```python
from build123d import *

# Parameters (mm, degrees)
SKETCH2_W                        = 90
SKETCH2_H                        = 90
BOSS_EXTRUDE1_DEPTH              = 103
SKETCH4_W                        = 24
SKETCH4_H                        = 25
SKETCH4_W_2                      = 40
SKETCH4_H_2                      = 17.5
SKETCH4_W_3                      = 3
SKETCH4_H_3                      = 4
SKETCH5_R                        = 10
CUT_EXTRUDE1_DEPTH               = 46
CUT_EXTRUDE1_DEPTH_BACK          = 46
SKETCH6_W                        = 87.169413833
SKETCH6_H                        = 43.101198191
CUT_EXTRUDE2_DEPTH               = 46
CUT_EXTRUDE2_DEPTH_BACK          = 46
CUT_EXTRUDE3_DEPTH               = 103
CUT_EXTRUDE4_REACH               = 92
SKETCH10_R                       = 1.7
FILLET1_R                        = 1
M16X1_5_TAPPED_HOLE2_D           = 14.5
M16X1_5_TAPPED_HOLE2_DEPTH       = 20
M16X1_5_TAPPED_HOLE2_CSINK_D     = 16.05
M16X1_5_TAPPED_HOLE2_CSINK_ANGLE = 90
M16X1_5_TAPPED_HOLE2_TIP         = 4.356239488
CIRPATTERN2_COUNT                = 4


with BuildPart() as part:
    # Sketch2 → Boss-Extrude1 (new body)
    with BuildSketch(Plane.XY):
        Rectangle(SKETCH2_W, SKETCH2_H)
    extrude(amount=BOSS_EXTRUDE1_DEPTH)

    # Sketch4 → Cut-Revolve2 (revolve, cut)
    with BuildSketch(Plane(origin=(0, 0, 0), x_dir=(1, 0, 0), z_dir=(0, 1, 0))):
        with Locations((12, -12.5)):
            Rectangle(SKETCH4_W, SKETCH4_H)
        Polygon((0, -25), (0, -39.420654857), (24, -25), align=None)
        with Locations((50, -8.75)):
            Rectangle(SKETCH4_W_2, SKETCH4_H_2)
        with Locations((28.5, -4.5)):
            Rectangle(SKETCH4_W_3, SKETCH4_H_3)
    revolve(axis=Axis((0, 0, 0), (0, 0, 1)), mode=Mode.SUBTRACT)

    # Sketch5 → Cut-Extrude1 (cut, two sides)
    with BuildSketch(Plane(origin=(0, 0, 0), x_dir=(0, 0, -1), z_dir=(1, 0, 0))) as cut_extrude1_sk:
        with Locations((-77.5, 0)):
            Circle(SKETCH5_R)
    extrude(amount=CUT_EXTRUDE1_DEPTH, mode=Mode.SUBTRACT)
    extrude(cut_extrude1_sk.sketch, amount=-CUT_EXTRUDE1_DEPTH_BACK, mode=Mode.SUBTRACT)

    # Sketch6 → Cut-Revolve3 (revolve, cut)
    with BuildSketch(Plane(origin=(0, 0, 0), x_dir=(0, 0, -1), z_dir=(1, 0, 0))):
        with Locations((-91.084706917, 51.550599096)):
            Rectangle(SKETCH6_W, SKETCH6_H)
    revolve(axis=Axis((0, 0, 0), (0, 0, 1)), mode=Mode.SUBTRACT)

    # Sketch7 → Cut-Extrude2 (cut, two sides)
    with BuildSketch(Plane(origin=(0, 0, 0), x_dir=(0, 0, -1), z_dir=(1, 0, 0))) as cut_extrude2_sk:
        with BuildLine():
            Line((-103, 30), (-103, 0))
            ThreePointArc((-103, 0), (-95.748626332, 19.557607216), (-77.5, 29.6605799))
            Line((-77.5, 29.6605799), (-77.5, 30))
            Line((-77.5, 30), (-103, 30))
        make_face()
        with BuildLine():
            ThreePointArc((-77.5, -29.6605799), (-95.748626332, -19.557607216), (-103, 0))
            Line((-103, 0), (-103, -30))
            Line((-103, -30), (-77.5, -30))
            Line((-77.5, -30), (-77.5, -29.6605799))
        make_face()
    extrude(amount=CUT_EXTRUDE2_DEPTH, mode=Mode.SUBTRACT)
    extrude(cut_extrude2_sk.sketch, amount=-CUT_EXTRUDE2_DEPTH_BACK, mode=Mode.SUBTRACT)

    # Sketch8 → Cut-Extrude3 (cut)
    with BuildSketch(Plane.XY.offset(47.5)):
        with BuildLine():
            ThreePointArc((30, 0), (28.722813233, 8.660254038), (25, 16.583123952))
            Line((25, 16.583123952), (25, -16.583123952))
            ThreePointArc((25, -16.583123952), (28.722813233, -8.660254038), (30, 0))
        make_face()
        with BuildLine():
            Line((-25, -16.583123952), (-25, 16.583123952))
            ThreePointArc((-25, 16.583123952), (-30, 0), (-25, -16.583123952))
        make_face()
        with BuildLine():
            ThreePointArc((10, 28.284271247), (0, 30), (-10, 28.284271247))
            Line((-10, 28.284271247), (-10, -28.284271247))
            ThreePointArc((-10, -28.284271247), (0, -30), (10, -28.284271247))
            Line((10, -28.284271247), (10, 28.284271247))
        make_face()
    extrude(amount=CUT_EXTRUDE3_DEPTH, mode=Mode.SUBTRACT)

    # Sketch10 → Cut-Extrude4 (cut, up to next)
    with BuildSketch(Plane(origin=(0, 45, 0), x_dir=(1, 0, 0), z_dir=(0, 1, 0)), mode=Mode.PRIVATE) as cut_extrude4_sk1:
        with Locations((0, -32.5)):
            Circle(SKETCH10_R)
    cut_extrude4_tool1 = extrude(cut_extrude4_sk1.sketch, amount=-CUT_EXTRUDE4_REACH, mode=Mode.PRIVATE) & part.part
    add(cut_extrude4_tool1.solids().sort_by_distance((0, 45, 32.5))[0], mode=Mode.SUBTRACT)

    # Fillet1
    fillet1_edges = [part.edges().sort_by_distance(p)[0] for p in [
        (18.452078799, 23.654191764, 47.5),
        (18.452078799, -23.654191764, 47.5),
        (-18.452078799, -23.654191764, 47.5),
        (25, 0, 47.5),
        (-25, 0, 47.5),
        (-10, 0, 47.5),
        (10, 0, 47.5),
        (-30, 0, 17.5),
        (-18.452078799, 23.654191764, 47.5),
    ]]
    fillet(fillet1_edges, radius=FILLET1_R)

    # M16x1.5 Tapped Hole2
    with Locations(Plane(origin=(0, 45, 0), x_dir=(1, 0, 0), z_dir=(0, 1, 0))):
        with Locations((0, -32.5)):
            CounterSinkHole(M16X1_5_TAPPED_HOLE2_D / 2, M16X1_5_TAPPED_HOLE2_CSINK_D / 2, depth=M16X1_5_TAPPED_HOLE2_DEPTH, counter_sink_angle=M16X1_5_TAPPED_HOLE2_CSINK_ANGLE)
            with Locations((0, 0, -(M16X1_5_TAPPED_HOLE2_DEPTH + M16X1_5_TAPPED_HOLE2_TIP / 2))):  # 118° drill point
                Cone(0, M16X1_5_TAPPED_HOLE2_D / 2, M16X1_5_TAPPED_HOLE2_TIP, mode=Mode.SUBTRACT)

    # Sketch25 → M12x1.5 Tapped Hole1 (revolve, cut)
    with BuildSketch(Plane(origin=(31.819805153, 31.819805153, 17.5), x_dir=(0, 1, 0), z_dir=(1, 0, 0))):
        Polygon((0, 0), (0, 23.15451825), (5.25, 20), (5.25, 0.775), (6.025, 0), align=None)
    m12x1_5_tapped_hole1 = revolve(axis=Axis((31.819805153, 31.819805153, 11.15), (0, 0, 1)), mode=Mode.SUBTRACT)

    # CirPattern2: M12x1.5 Tapped Hole1 ×4 about axis
    cirpattern2_axis = Axis((0, 0, 0), (0, 0, 1))
    for i in range(1, CIRPATTERN2_COUNT):
        add(m12x1_5_tapped_hole1.rotate(cirpattern2_axis, i * 360 / CIRPATTERN2_COUNT), mode=Mode.SUBTRACT)


solid = part.part
```
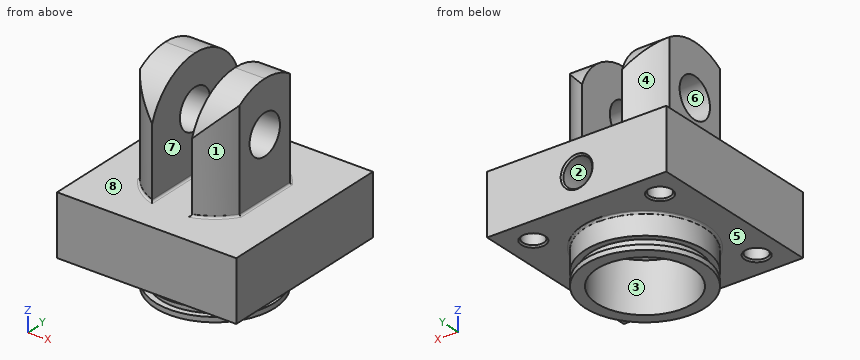
CAD build for the part. Positions are in the model's coordinates, mm. Face numbers are marked on the shaded views. A direction names the side the tool comes from. Round coordinates to 2 decimals unless told otherwise and drop trailing zeros. Order: outer loops, then holes, each group sorted by start corner. A loop starts at its lowest first (then second) coordinate and runs counter-clockwise, first axis right, second up. Notation, with made-up numbers: (5, 65) -> (52, 65) arc R3 cw to (52, 70) -> close; hole circle Ø7 at (76.25, 84.5). An arc over 180 degrees is marked (long way). One line per question, with ' | ' between items.
Q1. Slice it at B-B (z = 66). Write the cut outline in (x, y).
Completed:
outline: (-25, -16.58) arc R30 ccw to (-10, -28.28) -> (-10, 28.28) arc R30 ccw to (-25, 16.58) -> close; (10, -28.28) arc R30 ccw to (25, -16.58) -> (25, 16.58) arc R30 ccw to (10, 28.28) -> close
Q2. Probe probe 1 along Z at (x, y) = (-3.5, -27); probe 2 along X at (y, z) = (-25, 63.5); probe 3 along Z at (x, y) = (0, 13). List the from-to ranges inside material, lowest first.
Completed:
probe 1: z = 0 to 2.5, 6.5 to 47.5 | probe 2: x = -16.58 to -10, 10 to 16.58 | probe 3: z = 34.2 to 47.5
Q3. Which spindle directions (+Z, -Z, +X, -X, +Y, -Y) get a long thin tool onto all of the face, cutting with end or side? Do the marked faces 1, 2, 3 and 4. Say none if no direction does.
Completed:
face 1: +Z, +X, -Y | face 2: +Y | face 3: -Z | face 4: +Z, -X, +Y
Q4. Slice it at D-D (z = 32.5). Write the cut outline in (x, y) (3 decimals), then the cut area to 3 significant figures.
Completed:
outline: (-45, -45) -> (45, -45) -> (45, 45) -> (8.025, 45) -> (7.25, 44.225) -> (7.25, 25) -> (1.7, 21.665) -> (1.7, 11.392) arc R11.518 cw (long way) to (-1.7, 11.392) -> (-1.7, 21.665) -> (-7.25, 25) -> (-7.25, 44.225) -> (-8.025, 45) -> (-45, 45) -> close; hole circle Ø10.5 at (-31.82, -31.82); hole circle Ø10.5 at (-31.82, 31.82); hole circle Ø10.5 at (31.82, -31.82); hole circle Ø10.5 at (31.82, 31.82) | area: 6,980 mm^2
Q5. Two-plate mould, pull along Z, no slides. Class the marked faces 5, 6, 7 and 8: released by +Z, released by -Z, zero draft, split by the parting line, or undercut.
Completed:
face 5: released by -Z | face 6: undercut | face 7: zero draft | face 8: released by +Z
Q6. Slice it at A-A (z = 77.5). Write the cut outline in (x, y), then the cut area to 3 significant figures.
Completed:
outline: (-25, -16.58) arc R30 ccw to (-10, -28.28) -> (-10, -10) -> (-25, -10) -> close; (-25, 10) -> (-10, 10) -> (-10, 28.28) arc R30 ccw to (-25, 16.58) -> close; (10, -28.28) arc R30 ccw to (25, -16.58) -> (25, -10) -> (10, -10) -> close; (10, 10) -> (25, 10) -> (25, 16.58) arc R30 ccw to (10, 28.28) -> close | area: 825 mm^2
Q7. Drop flat-ended pins along their axis: pin 1 (17 mm diameter, centred on x = -31.82, y = 31.82, fed in from -Z); pin 2 (6 mm diameter, centred on x = -17.5, y = 27, fed in from +Z); pin 3 (12 mm diameter, centred on y = 0, z = 77.5, fed in from +X); pin 4 (10 mm diameter, centred on x = 29.5, z = 54.5, fed in from -Y). Give the stop position or say it passes through.
Completed:
pin 1: stops at z = 17.5 | pin 2: stops at z = 91 | pin 3: passes through | pin 4: stops at y = -17.31
Q8. Slice it at C-C (y = 5). Give the number of separate pieces and of enclosed holes in the cut face, then the cut area to 3 significant figures.
Completed:
separate pieces: 3 | enclosed holes: 0 | area: 3,370 mm^2
